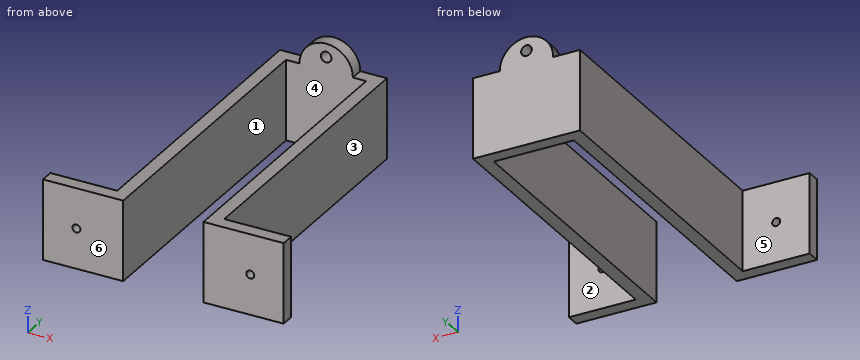
Autodesk Fusion 360 part; units mm, degrees
sketch "Boceto1" plane through (0, 0, 0) normal (0, 0, 1) x (1, 0, 0)
  line L0 (0, 0) -> (30, 0)
  line L1 (30, 0) -> (30, 110)
  line L2 (30, 110) -> (60, 110)
  line L3 (60, 110) -> (60, 0)
  line L4 (60, 0) -> (90, 0)
  line L5 (90, 0) -> (90, 5)
  line L6 (90, 5) -> (65, 5)
  line L7 (65, 5) -> (65, 115)
  line L8 (65, 115) -> (25, 115)
  line L9 (25, 115) -> (25, 5)
  line L10 (25, 5) -> (0, 5)
  line L11 (0, 5) -> (0, 0)
  dimension "d1" = 110
  dimension "d2" = 5
  dimension "d3" = 25
  dimension "d4" = 110
  dimension "d5" = 40
  dimension "d6" = 110
extrude "Extruir1" add sketch "Boceto1" along normal blind 30
sketch "Boceto2" plane through (0, 115, 0) normal (0, 1, 0) x (-1, 0, 0)
  line L0 (-65, 0) -> (-25, 0)
  line L1 (-25, 0) -> (-25, 30)
  line L2 (-25, 30) -> (-65, 30)
  line L3 (-65, 30) -> (-65, 0)
  circle A0 centre (-45, 30) radius 10
extrude "Extruir2" add sketch "Boceto2" against normal blind 5 contours L2 A0 picked at (-42.135, 33.3571)
sketch "Boceto3" plane through (0, 115, 0) normal (0, 1, 0) x (-1, 0, 0)
  line L0 (-65, 0) -> (-25, 0)
  line L1 (-25, 0) -> (-25, 30)
  line L2 (-25, 30) -> (-35, 30)
  arc A0 (-35, 30) -> (-55, 30) centre (-45, 30) ccw
  line L3 (-55, 30) -> (-65, 30)
  line L4 (-65, 30) -> (-65, 0)
  line L5 (-45, 40) -> (-45, 35)
  circle A1 centre (-45, 35) radius 2
  dimension "d11" = 5
  dimension "d12" = 4
extrude "Extruir3" cut sketch "Boceto3" against normal blind 5 contours A1
sketch "Boceto4" plane through (0, 5, 0) normal (0, 1, 0) x (-1, 0, 0)
  line L0 (-25, 0) -> (0, 0)
  line L1 (0, 0) -> (0, 30)
  line L2 (0, 30) -> (-25, 30)
  line L3 (-25, 30) -> (-25, 0)
  line L4 (-25, 30) -> (0, 0)
  line L5 (0, 30) -> (-25, 0)
  line L6 (-65, 0) -> (-90, 30)
  line L7 (-90, 30) -> (-90, 0)
  line L8 (-90, 0) -> (-65, 30)
  circle A0 centre (-77.5, 15) radius 1.5
  circle A1 centre (-12.5, 15) radius 1.5
  dimension "d15" = 3
  dimension "d16" = 3
extrude "Extruir4" cut sketch "Boceto4" against normal blind 5 contours L4 L5 A1 | L4 L5 A1 | L4 L5 A1 | L4 L5 A1 | L6 L8 A0 | L6 L8 A0 | L6 L8 A0 | L6 L8 A0
Build history of the part. All positions in model axes, mm. Face numbers are marked on the shaded views. A direction names the side the tool comes from. Coordinates: 2 decimals unless noted, no trailing zeros. Write each loop counter-clockwise with the first axis right and the second up, starting at its lowest first coordinate (ties: lowest second). Pieces come first, ordered by that corner, then holes.
(1) Cut at C-C on x = 12.5. List the corners of the cut face in (y, z).
(2) Mould opens along X. For the marked faces 1, 2 and 3 say: pulls with the +X half, pulls with the -X half, needs draft (parallel to the pull), parting line crosses it, or undercut.
(3) Drill centre lines: line 1 (X direction, y = 2.15, z = 15); line 2 (X direction, y = 59.5, z = 21.5); line 3 (Z direction, x = 77.5, y = 1.45). Where is each one in solid material? Low to high.
(4) Cut at B-B on y = 75. List the corners of the cut face in (x, z).
(5) Cut at A-A on z = 15. List the corners of the cut face in (x, y), and give its area (3 significant figures).
(6) Pin check, flat tips, straight feed: pin 1 Ø24 at (y, z) = (62, 9.5) entering from -X; pin 2 Ø4.5 at (x, z) = (45, 35) entering from -Y; pin 3 Ø15 at (y, z) = (43, 15.5) entering from +X; pin 4 Ø2.5 at (x, z) = (12.5, 15) entering from -Y. Stop position of each tip, or through.
(7) Cut at D-D on x = 61.5. List the corners of the cut face in (y, z).
(8) 3-axis set-ups, long thin cutter, end or side, ignore diameter. For the marked faces 4, 5 and 6: which of +Z, -Z, +X, -X, +Y, -Y reach the whole face in a straight line?
Working result:
1. outline: (0, 0) - (5, 0) - (5, 13.5) - (0, 13.5) - close; (0, 16.5) - (5, 16.5) - (5, 30) - (0, 30) - close
2. face 1: undercut
2. face 2: needs draft
2. face 3: pulls with the +X half
3. line 1: x = 0 to 11, 14 to 30, 60 to 76, 79 to 90
3. line 2: x = 25 to 30, 60 to 65
3. line 3: z = 0 to 13.5, 16.5 to 30
4. outline: (25, 0) - (30, 0) - (30, 30) - (25, 30) - close; (60, 0) - (65, 0) - (65, 30) - (60, 30) - close
5. outline: (0, 0) - (11, 0) - (11, 5) - (0, 5) - close; (14, 0) - (30, 0) - (30, 110) - (60, 110) - (60, 0) - (76, 0) - (76, 5) - (65, 5) - (65, 115) - (25, 115) - (25, 5) - (14, 5) - close; (79, 0) - (90, 0) - (90, 5) - (79, 5) - close
5. area: 1,520 mm2
6. pin 1: stops at x = 25
6. pin 2: stops at y = 110
6. pin 3: stops at x = 65
6. pin 4: passes through
7. outline: (0, 0) - (115, 0) - (115, 30) - (0, 30) - close
8. face 4: +Z, -Z, -Y
8. face 5: +Z, -Z, -X, +Y
8. face 6: +Z, -Z, +X, -X, -Y
